Build history of the part. All positions in model axes, mm. A direction names the side the tool comes from. Round coordinates to 2 decimals unless told otherwise and drop trailing zeros. Write each loop counter-clockwise with the first axis right and the second up, starting at its lowest first coordinate (ties: lowest second). Pieces come first, ordered by that corner, then holes. Notation, with made-up numbers: (61.5, -13) -> (111.5, -13) arc R13 cw to (111.5, -6) -> close; hole circle Ø9 at (-24.75, 52.25). An arc over 180 degrees is marked (long way). Answer as CSV lines item,"result".
from build123d import *

# Parameters (mm, degrees)
SKETCH2_W               = 55
SKETCH2_H               = 55
SKETCH2_R               = 20
BOSS_EXTRUDE1_DEPTH     = 8.18
CUT_EXTRUDE1_REACH      = 63.892
CUT_EXTRUDE1_END_RADIUS = 5.47
SKETCH3_R               = 2


# Read off the part's stored shape, not the designer's step: Revolve2
with BuildPart() as part:
    # Revolve2 outline → Revolve2 (revolve)
    with BuildSketch(Plane.XY):
        Polygon((2.86451, -3.5), (2.36451, -4), (2.36451, -4.25), (3.06451, -4.25), (3.06451, -6.03), (0.25, -6.03), (0.25, -7.03), (20, -7.03), (20, 1.15), (11.01, 1.15), (11.01, 1.65), (8.65, 1.65), (8.65, 1.15), (7.97, 1.15), (7.97, 0), (5.47, 0), (5.47, -3.5), align=None)
    revolve(axis=Axis((0, 0, 0), (0, 1, 0)))

    # Sketch2 → Boss-Extrude1 (add)
    with BuildSketch(Plane(origin=(0, 1.15, 0), x_dir=(1, 0, 0), z_dir=(0, 1, 0))):
        Rectangle(SKETCH2_W, SKETCH2_H)
        Circle(SKETCH2_R, mode=Mode.SUBTRACT)
    extrude(amount=-BOSS_EXTRUDE1_DEPTH)

    # Cut-Extrude1: up to this cylinder (the profile starts outside it)
    cut_extrude1_end = Plane(origin=(0, -2.85, 0), z_dir=(0, 1, 0)) * Cylinder(CUT_EXTRUDE1_END_RADIUS, 139.724, mode=Mode.PRIVATE)
    # Sketch3 → Cut-Extrude1 (cut, up to the surface)
    with BuildSketch(Plane(origin=(27.5, 0, 0), x_dir=(0, 0, -1), z_dir=(1, 0, 0)), mode=Mode.PRIVATE) as cut_extrude1_sk1:
        with Locations((0, -2.85)):
            Circle(SKETCH3_R)
    cut_extrude1_tool1 = extrude(cut_extrude1_sk1.sketch, amount=-CUT_EXTRUDE1_REACH, mode=Mode.PRIVATE) - cut_extrude1_end
    add(cut_extrude1_tool1.solids().sort_by_distance((27.5, -2.85, 0))[0], mode=Mode.SUBTRACT)


solid = part.part
1. Drop flat-ended pins along their axis: pin 1 Ø17.5 at (x, z) = (-2, -3.5) entering from +Y; pin 2 Ø5.5 at (x, z) = (0.5, 2.5) entering from +Y; pin 3 Ø5.5 at (x, z) = (0, 0) entering from +Y. Give the stop position or say it passes through.
Results found:
pin 1,"stops at y = 1.65"
pin 2,"stops at y = -3.5"
pin 3,"stops at y = -3.61"
2. Cut at D-D, the plane x = -9.5. Write the cut outline in (y, z).
Results found:
outline,"(-7.03, -27.5) -> (1.15, -27.5) -> (1.15, -5.57) -> (1.65, -5.57) -> (1.65, 5.57) -> (1.15, 5.57) -> (1.15, 27.5) -> (-7.03, 27.5) -> close"
3. Probe line 1 along Z through (x, y) = (0, -4.05); line 2 along X through (y, z) = (-4.1, 0); line 3 along X through (y, z) = (-5.55, 0). List the from-to ranges inside material, lowest first.
Results found:
line 1,"z = -27.5 to -2.36, 2.36 to 27.5"
line 2,"x = -27.5 to -2.36, 2.36 to 5.47"
line 3,"x = -27.5 to -3.06, 3.06 to 27.5"
4. Cut at C-C, the plane z = -15. Write the cut outline in (x, y).
Results found:
outline,"(-27.5, -7.03) -> (27.5, -7.03) -> (27.5, 1.15) -> (-27.5, 1.15) -> close"
5. Cut at B-B, the plane y = -2.85. Write the cut outline in (x, z).
Results found:
outline,"(-27.5, -27.5) -> (27.5, -27.5) -> (27.5, -2) -> (5.09, -2) arc R5.47 cw (long way) to (5.09, 2) -> (27.5, 2) -> (27.5, 27.5) -> (-27.5, 27.5) -> close"
6. Cut at A-A, the plane x = 18. Write the cut outline in (y, z), then the cut area to 3 significant figures.
Results found:
outline,"(-7.03, -27.5) -> (1.15, -27.5) -> (1.15, 27.5) -> (-7.03, 27.5) -> close; hole circle Ø4 at (-2.85, 0)"
area,"437 mm2"
7. Mould opens along Y. For faces 4 (the flat face through (0, -3, -27.5)), 5 (the flat face through (-5.4, 0, 1.7)), 6 (the flat face through (-2, -4.25, 2)) say: +Y half, -Y half, draft (parallel to the pull), parting line (faces both ways), or undercut.
Results found:
face 4,"draft"
face 5,"+Y half"
face 6,"undercut"
8. Which spindle directions (+Z, -Z, +X, -X, +Y, -Y) get a long thin tool onto all of the face, cutting with end or side? Do faces 1 (the flat face through (2.4, -3.5, 2.4)), 2 (the cylindrical face through (16.452, -4.802, 0.434)), 3 (the cylindrical face through (-0.4, -5.15, -3.04)). Say none if no direction does.
Results found:
face 1,"+Y"
face 2,"+X"
face 3,"none"
